CAD build for the part. Positions are in the model's coordinates, mm. A direction names the side the tool comes from. Give positions to 0.01 mm unless a question says otherwise; leave off trailing zeros. Loops run counter-clockwise (first coordinate to the right, second up) from the corner with the lowest first, then second, coordinate; pieces in that order, holes last. Notation, with made-up numbers: M 52,42.5 L 64,42.5 A11 cw 64,54.5 Z; hole C 61.5,20 d6. An arc over 180 degrees is marked long. Answer as CSV lines item,"result".
from build123d import *

# Parameters (mm, degrees)
BOSS_EXTRUDE1_DEPTH = 3


with BuildPart() as part:
    # Sketch1 → Boss-Extrude1 (new body)
    with BuildSketch(Plane.XY):
        Polygon((-38, 40), (-38, 37.5), (-35, 37.5), (-35, 22.5), (-38, 22.5), (-38, 7.5), (-35, 7.5), (-35, -7.5), (-38, -7.5), (-38, -22.5), (-35, -22.5), (-35, -37.5), (-38, -37.5), (-38, -40), (-27.5, -40), (-27.5, -43), (-7.5, -43), (-7.5, -40), (7.5, -40), (7.5, -43), (27.5, -43), (27.5, -40), (38, -40), (38, -37.5), (35, -37.5), (35, -22.5), (38, -22.5), (38, -7.5), (35, -7.5), (35, 7.5), (38, 7.5), (38, 22.5), (35, 22.5), (35, 37.5), (38, 37.5), (38, 40), align=None)
        with BuildLine():
            Line((-12.5, 25), (-12.5, -25))
            ThreePointArc((-12.5, -25), (-17.5, -30), (-22.5, -25))
            Line((-22.5, -25), (-22.5, 25))
            ThreePointArc((-22.5, 25), (-17.5, 30), (-12.5, 25))
        make_face(mode=Mode.SUBTRACT)
        with BuildLine():
            ThreePointArc((5, -25), (0, -30), (-5, -25))
            Line((-5, -25), (-5, 25))
            ThreePointArc((-5, 25), (0, 30), (5, 25))
            Line((5, 25), (5, -25))
        make_face(mode=Mode.SUBTRACT)
        with BuildLine():
            ThreePointArc((22.5, -25), (17.5, -30), (12.5, -25))
            Line((12.5, -25), (12.5, 25))
            ThreePointArc((12.5, 25), (17.5, 30), (22.5, 25))
            Line((22.5, 25), (22.5, -25))
        make_face(mode=Mode.SUBTRACT)
    extrude(amount=BOSS_EXTRUDE1_DEPTH)


solid = part.part
1) Drill centre lines: line 1 (X direction, y = 2, z = 2); line 2 (X direction, y = 20.5, z = 0.5); line 3 (Y direction, x = 33.5, z = 1.1). Where is each one in solid material? Low to high. Write a range as from..to.
Answer below:
line 1,"x = -35..-22.5, -12.5..-5, 5..12.5, 22.5..35"
line 2,"x = -38..-22.5, -12.5..-5, 5..12.5, 22.5..38"
line 3,"y = -40..40"
2) Which spindle directions (+Z, -Z, +X, -X, +Y, -Y) get a long thin tool onto all of the face, cutting with end or side? Do faces 5 (the face through (36, -22.5, 1)), 6 (the face through (33, -40, 1)), 7 (the face through (-35, -30, 1)), 8 (the face through (-17.6, 30, 1.5)). Say none if no direction does.
Answer below:
face 5,"+Z, -Z, +X"
face 6,"+Z, -Z, +X, -Y"
face 7,"+Z, -Z, -X"
face 8,"+Z, -Z"
3) Band-saw the part on D-D on z = 0.95. Give the number of separate pieces and of enclosed holes in the cut face, and give its area (3 significant figures).
Answer below:
separate pieces,"1"
enclosed holes,"3"
area,"4,190 mm^2"
4) Band-saw the part on B-B on x = 0. Give the cut face in (y, z).
Answer below:
outline,"M -40,0 L -30,0 L -30,3 L -40,3 Z; M 30,0 L 40,0 L 40,3 L 30,3 Z"
5) Flat gauge pins, fed straight in: pin 1 (1.5 mm diameter, centred on x = -36, z = 2, fed in from -Y); pin 2 (0.9 mm diameter, centred on y = -41.5, z = 1, fed in from -X); pin 3 (1.5 mm diameter, centred on y = -29, z = 1.5, fed in from -X). Where does each tip first touch, or does it go through?
Answer below:
pin 1,"stops at y = -40"
pin 2,"stops at x = -27.5"
pin 3,"stops at x = -35"
6) Mould opens along Y. For faces 1 (the face through (-18, -43, 1)), 2 (the face through (-36, 22.5, 1)), 3 (the face through (22.5, 0, 1)), 4 (the face through (-27.5, -41, 1)) say: +Y half, -Y half, draft (parallel to the pull), parting line (faces both ways), or undercut.
Answer below:
face 1,"-Y half"
face 2,"undercut"
face 3,"undercut"
face 4,"draft"
7) Band-saw the part on A-A on y = 6. Give the cut face in (x, z).
Answer below:
outline,"M -35,0 L -22.5,0 L -22.5,3 L -35,3 Z; M -12.5,0 L -5,0 L -5,3 L -12.5,3 Z; M 5,0 L 12.5,0 L 12.5,3 L 5,3 Z; M 22.5,0 L 35,0 L 35,3 L 22.5,3 Z"
8) Band-saw the part on C-C on x = 17.5. Give the cut face in (y, z).
Answer below:
outline,"M -43,0 L -30,0 L -30,3 L -43,3 Z; M 30,0 L 40,0 L 40,3 L 30,3 Z"
